```python
from build123d import *

# Parameters (mm, degrees)
F1_DEPTH = 9.525
F2_R     = 1.905
F3_R     = 1.016
F4_R     = 2.54


with BuildPart() as f1:
    # F0 (on Top) → F1 (new body)
    with BuildSketch(Plane.XY):
        Polygon((-3.175, 16.309805), (-3.175, -16.08006), (42.799, -11.659483), (42.799, 11.889228), align=None)
        Polygon((39.624, -8.775128), (0, -12.585128), (0, 12.814872), (39.624, 9.004872), align=None, mode=Mode.SUBTRACT)
    extrude(amount=F1_DEPTH)

    # F2
    f2_edges = [f1.edges().sort_by_distance(p)[0] for p in [
        (42.799, -11.659483, 4.7625),
        (42.799, 11.889228, 4.7625),
        (-3.175, 16.309805, 4.7625),
        (-3.175, -16.08006, 4.7625),
    ]]
    fillet(f2_edges, radius=F2_R)

    # F3
    f3_edges = [f1.edges().sort_by_distance(p)[0] for p in [
        (0, 12.814872, 4.7625),
        (0, -12.585128, 4.7625),
    ]]
    fillet(f3_edges, radius=F3_R)

    # F4
    f4_edges = [f1.edges().sort_by_distance(p)[0] for p in [
        (39.624, 9.004872, 4.7625),
        (39.624, -8.775128, 4.7625),
    ]]
    fillet(f4_edges, radius=F4_R)


solid = f1.part
```
Verification items for the finished model (mm, model axes). A direction names the side the tool comes from. Give positions to 0.01 mm unless a question says otherwise; leave off trailing zeros. Order: outer loops, then holes, each group sorted by start corner. A loop starts at its lowest first (then second) coordinate and runs counter-clockwise, first axis right, second up. Notation, with made-up numbers: (41, -29) - (79, -29) arc R6 cw to (79, -24) - close; hole circle Ø8 at (57, 25). An arc over 180 degrees is marked (long way). Answer as CSV lines item,"result". Start each with the question number.
Item 1: Material ranges on L1, parallel to X at y = -5.5, z = 9 (3 decimals); L2, parallel to Y at x = 17, z = 2.5; L3, parallel to Y at x = 31.5, z = 3.5, recorded low to high.
Item 2: Section check D-D, the plane y = -13. Record the boundary of the cut face in (x, z) (3 decimals).
Item 3: Access from +Z, -Z, +X, -X, +Y, -Y to the whole of each face (thin tool, end or side, straight path). Record for faces 4 (the face through (42.291, 11.454, 4.829)), 5 (the face through (38.95, 8.42, 4.83)).
Item 4: Section check A-A, the plane y = 2.5. Record the boundary of the cut face in (x, z) (3 decimals).
Item 5: Section check B-B, the plane z = 3.25. Record the boundary of the cut face in (x, y) (1 decimal), plus the area to 3 significant figures.
Item 6: Gauge pin test, flat ends, axial feed: pin 1 (3 mm diameter, centred on x = 28.5, z = 7.5, fed in from -Y); pin 2 (12 mm diameter, centred on x = 10.5, y = -2, fed in from -Z); pin 3 (5 mm diameter, centred on x = 24, z = 7, fed in from -Y). Record the tip position at first contact, or that the pin passes through.
Item 7: Mould release check, pull along X, two halves, no side actions. Record for faces 1 (the face through (18.97, 10.99, 4.7)), 2 (the face through (-3.175, 0, 5)), 3 (the face through (42.291, -11.224, 4.829)): released by +X, released by -X, zero draft, split by the parting line, or undercut.
Item 8: Section check C-C, the plane x = 8. Record the boundary of the cut face in (y, z) (3 decimals), plus the area to 3 significant figures.
Filled in:
1,L1,"-3.175 to 0, 39.624 to 42.799"
1,L2,"-14.14 to -10.95, 11.18 to 14.37"
1,L3,"-12.75 to -9.56, 9.79 to 12.98"
2,outline,"(-3.175, 0) - (28.858, 0) - (28.858, 9.525) - (-3.175, 9.525) - close"
3,face 4,"+Z, -Z, +X, +Y"
3,face 5,"+Z, -Z"
4,outline,"(-3.175, 0) - (0, 0) - (0, 9.525) - (-3.175, 9.525) - close; (39.624, 0) - (42.799, 0) - (42.799, 9.525) - (39.624, 9.525) - close"
5,outline,"(-3.2, -14) arc R1.9 ccw to (-1.1, -15.9) - (41.1, -11.8) arc R1.9 ccw to (42.8, -9.9) - (42.8, 10.2) arc R1.9 ccw to (41.1, 12.1) - (-1.1, 16.1) arc R1.9 ccw to (-3.2, 14.2) - close; hole (0, -11.5) arc R1 ccw to (1.1, -12.5) - (37.3, -9) arc R2.5 ccw to (39.6, -6.5) - (39.6, 6.7) arc R2.5 ccw to (37.3, 9.2) - (1.1, 12.7) arc R1 ccw to (0, 11.7) - close"
5,area,"430 mm^2"
6,pin 1,"y = -13.18"
6,pin 2,"through"
6,pin 3,"y = -13.71"
7,face 1,"undercut"
7,face 2,"released by -X"
7,face 3,"released by +X"
8,outline,"(-15.006, 0) - (-11.816, 0) - (-11.816, 9.525) - (-15.006, 9.525) - close; (12.046, 0) - (15.235, 0) - (15.235, 9.525) - (12.046, 9.525) - close"
8,area,"60.8 mm^2"
